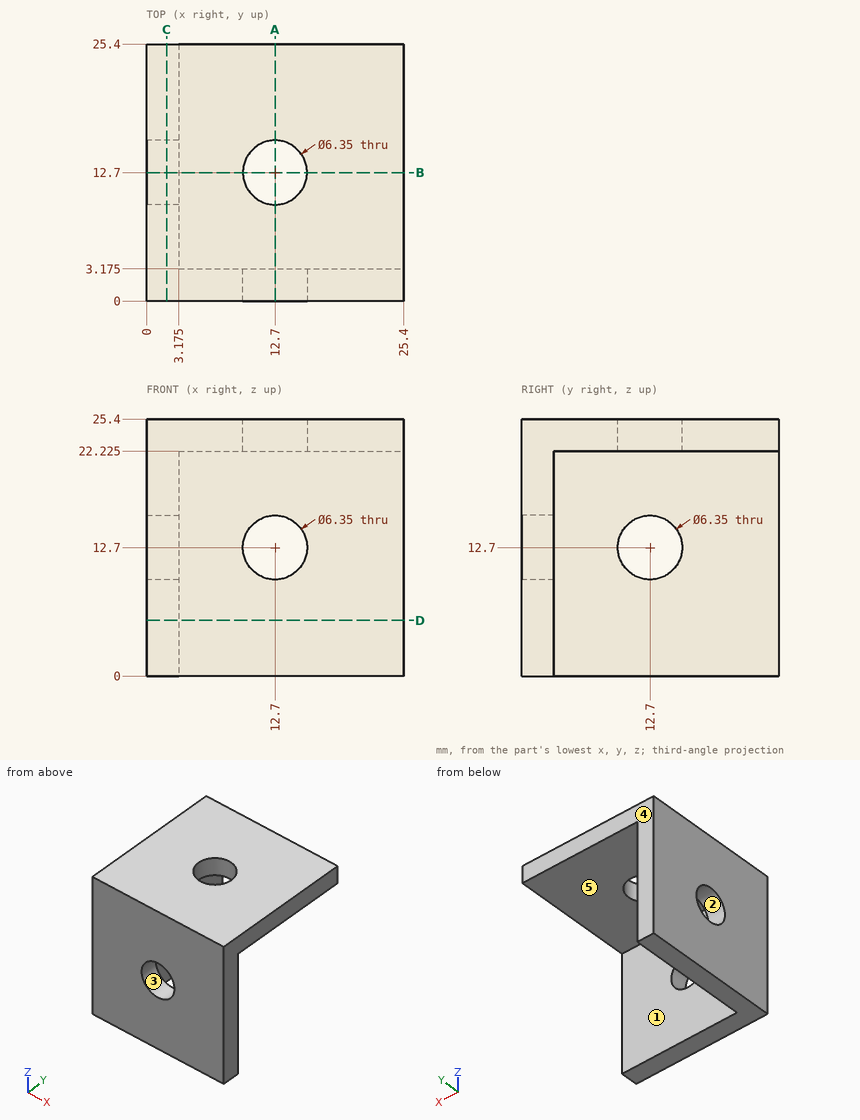
Here's the drawing with two shaded views (mm, measured from the low corner). I have some questions. A direction names the side the tool comes from. Round coordinates to 2 decimals unless told otherwise and drop trailing zeros. Write each loop counter-clockwise with the first axis right and the second up, starting at its lowest first coordinate (ties: lowest second). Pieces come first, ordered by that corner, then holes. Notation, with made-up numbers: M 2,79.25 L 51,79.25 A26 ccw 51,99.25 Z; hole C -25,77.25 d6. An arc over 180 degrees is marked long. Use CSV: the item, a comma, the result in double quotes.
(1) Imagine slicing it at A-A (x = 12.7). Write out the boundary of the cut face in (y, z) (3 decimals).
Check values:
outline,"M 0,0 L 3.175,0 L 3.175,9.525 L 0,9.525 Z; M 0,15.875 L 3.175,15.875 L 3.175,22.225 L 9.525,22.225 L 9.525,25.4 L 0,25.4 Z; M 15.875,22.225 L 25.4,22.225 L 25.4,25.4 L 15.875,25.4 Z"
(2) Imagine slicing it at D-D (z = 5.5). Write out the boundary of the cut face in (x, y) (3 decimals).
Check values:
outline,"M 0,0 L 25.4,0 L 25.4,3.175 L 3.175,3.175 L 3.175,25.4 L 0,25.4 Z"
(3) Imagine slicing it at C-C (x = 2). Write out the boundary of the cut face in (y, z) (3 decimals), plus the area to 3 significant figures.
Check values:
outline,"M 0,0 L 25.4,0 L 25.4,25.4 L 0,25.4 Z; hole C 12.7,12.7 d6.35"
area,"613 mm^2"
(4) We'd pull the mould along Y, two halves only. Please class the marked faces 1, 2 and 3: +Y half, -Y half, draft (parallel to the pull), parting line (faces both ways), or undercut.
Check values:
face 1,"+Y half"
face 2,"undercut"
face 3,"draft"
(5) I'm going to push flat-ended pins straight in: pin 1 (12 mm diameter, centred on x = 10.5, y = 12, fed in from -Z) (3 decimals); pin 2 (6 mm diameter, centred on y = 10.5, z = 6.5, fed in from +X) (3 decimals); pin 3 (3 mm diameter, centred on x = 19.5, z = 10, fed in from +Y) (3 decimals); pin 4 (5 mm diameter, centred on y = 12.7, z = 12.7, fed in from -X). Where does each tip first touch, or does it pass through?
Check values:
pin 1,"z = 22.225"
pin 2,"x = 3.175"
pin 3,"y = 3.175"
pin 4,"through"
(6) On a 3-axis mill with a long thin cutter (end or side, diameter ignored), from which of +Z, -Z, +X, -X, +Y, -Y can I reach the whole of each face in a straight line? I mean the marked faces 4 and 5. Say none if no direction works.
Check values:
face 4,"+Z, -Z, +X, -X, +Y"
face 5,"-Z, +X, +Y"
(7) I need wall thicknesses on line 1 along Y through (x, z) = (0.8, 12.7) (3 decimals); line 2 along Y through (x, z) = (19.5, 18.5) (3 decimals). Which ranges of each line are inside material? Lowest first, please.
Check values:
line 1,"0 to 9.525, 15.875 to 25.4"
line 2,"0 to 3.175"
